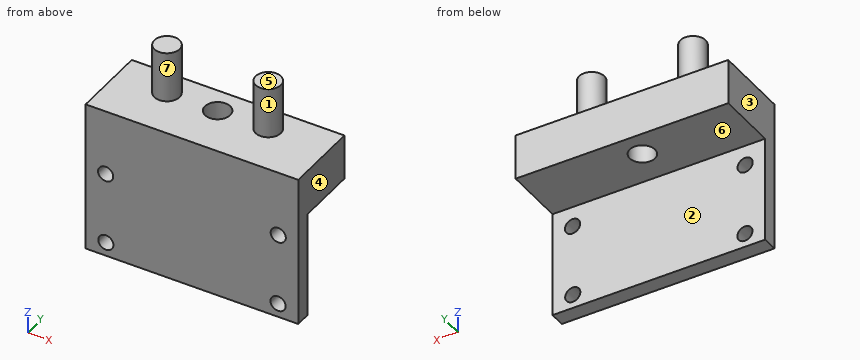
```python
from build123d import *

# Parameters (mm, degrees)
SKETCH1_W           = 42
SKETCH1_H           = 21
SKETCH1_R           = 1.5
BOSS_EXTRUDE1_DEPTH = 3
SKETCH1_3_W         = 42
SKETCH1_3_H         = 9
BOSS_EXTRUDE2_DEPTH = 15
SKETCH2_R           = 2.5
BOSS_EXTRUDE3_DEPTH = 10
SKETCH2_4_R         = 2.5
CUT_EXTRUDE2_DEPTH  = 10


with BuildPart() as part:
    # Sketch1 → Boss-Extrude1 (new body)
    with BuildSketch(Plane(origin=(0, 0, 0), x_dir=(1, 0, 0), z_dir=(0, 1, 0))):
        with Locations((0, 4.5)):
            Rectangle(SKETCH1_W, SKETCH1_H)
        with Locations((-17.044088176, -2)):
            Circle(SKETCH1_R, mode=Mode.SUBTRACT)
        with Locations((17.044088176, -2)):
            Circle(SKETCH1_R, mode=Mode.SUBTRACT)
        with Locations((-17, 12.248496994)):
            Circle(SKETCH1_R, mode=Mode.SUBTRACT)
        with Locations((17, 12.248496994)):
            Circle(SKETCH1_R, mode=Mode.SUBTRACT)
    extrude(amount=BOSS_EXTRUDE1_DEPTH)

    # Sketch1<3> → Boss-Extrude2 (add)
    with BuildSketch(Plane(origin=(0, 0, 0), x_dir=(1, 0, 0), z_dir=(0, 1, 0))):
        with Locations((0, -10.5)):
            Rectangle(SKETCH1_3_W, SKETCH1_3_H)
    extrude(amount=BOSS_EXTRUDE2_DEPTH)

    # Sketch2 → Boss-Extrude3 (add)
    with BuildSketch(Plane.XY.offset(15)):
        with Locations((9, 10)):
            Circle(SKETCH2_R)
        with Locations((-11, 10)):
            Circle(SKETCH2_R)
    extrude(amount=BOSS_EXTRUDE3_DEPTH)

    # Sketch2<4> → Cut-Extrude2 (cut)
    with BuildSketch(Plane.XY.offset(15)):
        with Locations((-1, 10)):
            Circle(SKETCH2_4_R)
    extrude(amount=-CUT_EXTRUDE2_DEPTH, mode=Mode.SUBTRACT)


solid = part.part
```
Part model, mm, in its own coordinate system. Face numbers are marked on the shaded views. A direction names the side the tool comes from. Round coordinates to 2 decimals unless told otherwise and drop trailing zeros. Order: outer loops, then holes, each group sorted by start corner. A loop starts at its lowest first (then second) coordinate and runs counter-clockwise, first axis right, second up. Notation, with made-up numbers: M 80.25,85.25 L 111.25,85.25 A14 cw 111.25,103.25 Z; hole C 33.5,-15.5 d9. An arc over 180 degrees is marked long. Put each result on its own line as item: value. Start each with the question number.
1. Drill centre lines: probe 1 along Y at (x, z) = (-1, 8.75); probe 2 along Y at (x, z) = (-15, 0); probe 3 along Z at (x, y) = (5.5, 12). Where is each one in solid material? Low to high. Write a range as [from, to].
2. Slice it at A-A on y = 10. List the corners of the cut face in (x, z).
3. Tool access for the marked faces 5, 6 and 7: list every direction of +Z, -Z, +X, -X, +Y, -Y with a clear straight run to the whole face (end or side of a thin tool).
4. Slice it at B-B on x = -3. List the corners of the cut face in (y, z), then the cut area to 3 significant figures.
5. Slice it at C-C on z = 6.5. List the corners of the cut face in (x, y), then the cut area to 3 significant figures.
6. Drop flat-ended pins along their axis: pin 1 (6.5 mm diameter, centred on x = -5.5, z = -8, fed in from +Y); pin 2 (2.5 mm diameter, centred on x = -17, z = -12.25, fed in from +Y); pin 3 (7.5 mm diameter, centred on x = -4.5, y = 4, fed in from +Z); pin 4 (6 mm diameter, centred on x = -10.5, y = 10.5, fed in from -Z). Give the stop position or say it passes through.
7. Slice it at D-D on x = -15. List the corners of the cut face in (y, z).
8. Two-plate mould, pull along X, no slides. Class the marked faces 1, 2, 3 and 4: +X half, -X half, draft (parallel to the pull), parting line (faces both ways), or undercut.
Findings:
1. probe 1: [0, 7.5], [12.5, 15]
1. probe 2: [0, 3]
1. probe 3: [6, 15]
2. outline: M -21,6 L -3.5,6 L -3.5,15 L -8.5,15 L -8.5,25 L -13.5,25 L -13.5,15 L -21,15 Z; M 1.5,6 L 21,6 L 21,15 L 11.5,15 L 11.5,25 L 6.5,25 L 6.5,15 L 1.5,15 Z
3. face 5: +Z, +X, -X, +Y, -Y
3. face 6: -Z, +X, -X, +Y
3. face 7: +Z
4. outline: M 0,-15 L 3,-15 L 3,6 L 8.5,6 L 8.5,15 L 0,15 Z; M 11.5,6 L 15,6 L 15,15 L 11.5,15 Z
4. area: 171 mm2
5. outline: M -21,0 L 21,0 L 21,15 L -21,15 Z; hole C -1,10 d5
5. area: 610 mm2
6. pin 1: y = 3
6. pin 2: through
6. pin 3: z = 15
6. pin 4: z = 6
7. outline: M 0,-15 L 3,-15 L 3,6 L 15,6 L 15,15 L 0,15 Z
8. face 1: undercut
8. face 2: draft
8. face 3: -X half
8. face 4: +X half
